Here's how the part is built. I have some questions about the finished solid (model axes, mm). Face numbers are marked on the shaded views. A direction names the side the tool comes from. Round coordinates to 2 decimals unless told otherwise and drop trailing zeros. Write each loop counter-clockwise with the first axis right and the second up, starting at its lowest first coordinate (ties: lowest second). Pieces come first, ordered by that corner, then holes. Notation, with made-up numbers: (7, 81) - (45, 81) arc R24 cw to (45, 119) - close; hole circle Ø6 at (-8.75, 80.25). An arc over 180 degrees is marked (long way). One line per item, written item: value. Start each with the question number.
Item 1: Thinking about a two-plate mould opening in X: for the marked faces 3, 4 and 5, which applies, released by +X, released by -X, zero draft, split by the parting line, or undercut?
Item 2: Imagine slicing it at C-C, the plane y = -70. Please give me the cut outline in (x, z), then the cut area to 3 significant figures.
Item 3: Imagine slicing it at B-B, the plane z = -74.5. Please give me the cut outline in (x, y).
Item 4: Imagine slicing it at D-D, the plane z = -63. Please give me the cut outline in (x, y), then the cut area to 3 significant figures.
Item 5: For P1, Ø3.5, axis at y = 11.5, z = -28.5, coming from the -X side; P2, Ø3, axis at x = 11.5, y = -166.5, coming from the +Z side; P3, Ø3.5, axis at y = 15.27, z = -50, coming from the +X side; P4, Ø8, axis at x = 19.5, z = -19.5, coming from the +Y side, each with a flat end and sliding along its axis, tell me the tip position at first contact or that it passes through.
Item 6: For the marked faces 1 and 2, which set-ups out of +Z, -Z, +X, -X, +Y, -Y let a thin tool reach every point of the face, with its end or its side?
Item 7: Imagine slicing it at A-A, the plane z = -39. Please give me the cut outline in (x, y).
Item 8: If I drill on line 1 (X direction, y = -7, z = -71); line 2 (X direction, y = -242.6, z = -4.5); line 3 (X direction, y = -131.5, z = -14), over which ranges is the centre line in solid material (lowest first)?
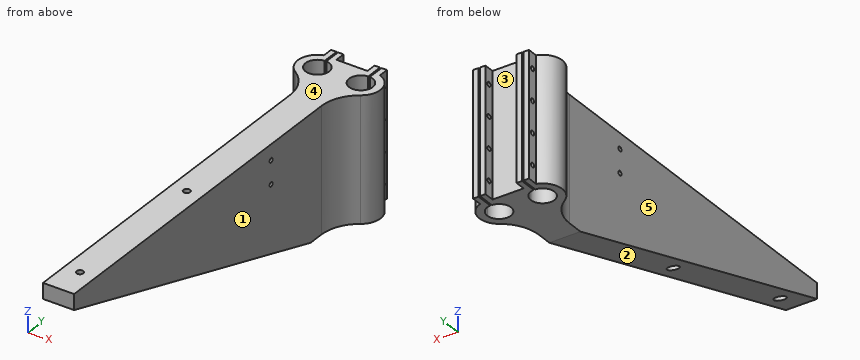
```python
from build123d import *

# Parameters (mm, degrees)
F0_R      = 7.6
F1_DEPTH  = 80
F2_DEPTH  = 80
F3_R      = 2.15
F4_DEPTH  = 80.001
F5_R      = 3.65
F6_DEPTH  = 70
F8_DEPTH  = 36.601
F9_W      = 0.5
F9_H      = 18.6
F10_DEPTH = 80.001
F11_R     = 1.45
F12_DEPTH = 44.601
F13_R     = 1.45
F14_DEPTH = 36.601


with BuildPart() as f1:
    # F0 (on Top) → F1 (new body)
    with BuildSketch(Plane.XY):
        with BuildLine():
            Line((-4, 18.6), (-4, 11.948222))
            ThreePointArc((-4, 11.948222), (-12.485747, 1.692961), (-7.037234, -10.451667))
            ThreePointArc((-7.037234, -10.451667), (1.06886, -19.443232), (4, -31.189101))
            Line((4, -31.189101), (4, -262.6))
            Line((4, -262.6), (24, -262.6))
            Line((24, -262.6), (24, -31.189101))
            ThreePointArc((24, -31.189101), (26.93114, -19.443232), (35.037234, -10.451667))
            ThreePointArc((35.037234, -10.451667), (40.485747, 1.692961), (32, 11.948222))
            Line((32, 11.948222), (32, 18.6))
            Line((32, 18.6), (24, 18.6))
            Line((24, 18.6), (24, 11.948222))
            Line((24, 11.948222), (4, 11.948222))
            Line((4, 11.948222), (4, 18.6))
            Line((4, 18.6), (-4, 18.6))
        make_face()
        Circle(F0_R, mode=Mode.SUBTRACT)
        with Locations((28, 0)):
            Circle(F0_R, mode=Mode.SUBTRACT)
    extrude(amount=-F1_DEPTH)

    # F0 (on Top) → F2 (join)
    with BuildSketch(Plane.XY):
        with BuildLine():
            Line((-4, 18.6), (-4, 11.948222))
            ThreePointArc((-4, 11.948222), (-12.485747, 1.692961), (-7.037234, -10.451667))
            ThreePointArc((-7.037234, -10.451667), (1.06886, -19.443232), (4, -31.189101))
            Line((4, -31.189101), (4, -262.6))
            Line((4, -262.6), (24, -262.6))
            Line((24, -262.6), (24, -31.189101))
            ThreePointArc((24, -31.189101), (26.93114, -19.443232), (35.037234, -10.451667))
            ThreePointArc((35.037234, -10.451667), (40.485747, 1.692961), (32, 11.948222))
            Line((32, 11.948222), (32, 18.6))
            Line((32, 18.6), (24, 18.6))
            Line((24, 18.6), (24, 11.948222))
            Line((24, 11.948222), (4, 11.948222))
            Line((4, 11.948222), (4, 18.6))
            Line((4, 18.6), (-4, 18.6))
        make_face()
        Circle(F0_R, mode=Mode.SUBTRACT)
        with Locations((28, 0)):
            Circle(F0_R, mode=Mode.SUBTRACT)
    extrude(amount=-F2_DEPTH)

    # F3 (on face) → F4 (cut, through all)
    with BuildSketch(Plane.XY):
        with Locations((14, -142.6)):
            Circle(F3_R)
        with Locations((14, -242.6)):
            Circle(F3_R)
    extrude(amount=-F4_DEPTH, mode=Mode.SUBTRACT)

    # F5 (on face) → F6 (cut)
    with BuildSketch(Plane(origin=(0, 0, -80), x_dir=(1, 0, 0), z_dir=(0, 0, -1))):
        with Locations((14, 242.6)):
            Circle(F5_R)
        with Locations((14, 142.6)):
            Circle(F5_R)
    extrude(amount=-F6_DEPTH, mode=Mode.SUBTRACT)

    # F7 (on face) → F8 (cut, through all)
    with BuildSketch(Plane(origin=(4, 0, 0), x_dir=(0, -1, 0), z_dir=(-1, 0, 0))):
        Polygon((262.6, -80), (262.6, -10), (41.189101, -80), align=None)
    extrude(amount=-F8_DEPTH, mode=Mode.SUBTRACT)

    # F9 (on face) → F10 (cut, through all)
    with BuildSketch(Plane.XY):
        with Locations((-0.25, 9.3)):
            Rectangle(F9_W, F9_H)
        with Locations((0.25, 9.3)):
            Rectangle(F9_W, F9_H)
        with Locations((27.75, 9.3)):
            Rectangle(F9_W, F9_H)
        with Locations((28.25, 9.3)):
            Rectangle(F9_W, F9_H)
    extrude(amount=-F10_DEPTH, mode=Mode.SUBTRACT)

    # F11 (on face) → F12 (cut, through all)
    with BuildSketch(Plane(origin=(-4, 0, 0), x_dir=(0, -1, 0), z_dir=(-1, 0, 0))):
        with Locations((-15.274111, -30)):
            Circle(F11_R)
        with Locations((-15.274111, -70)):
            Circle(F11_R)
        with Locations((-15.274111, -50)):
            Circle(F11_R)
        with Locations((-15.274111, -10)):
            Circle(F11_R)
    extrude(amount=-F12_DEPTH, mode=Mode.SUBTRACT)

    # F13 (on face) → F14 (cut, through all)
    with BuildSketch(Plane(origin=(4, 0, 0), x_dir=(0, -1, 0), z_dir=(-1, 0, 0))):
        with Locations((78.189101, -10)):
            Circle(F13_R)
        with Locations((78.189101, -25)):
            Circle(F13_R)
    extrude(amount=-F14_DEPTH, mode=Mode.SUBTRACT)


solid = f1.part
```
Values follow:
1. face 3: undercut
1. face 4: zero draft
1. face 5: released by -X
2. outline: (4, -70.89) - (24, -70.89) - (24, 0) - (4, 0) - close
2. area: 1,420 mm^2
3. outline: (-7.04, -10.45) arc R25 cw to (4, -31.19) - (4, -58.59) - (24, -58.59) - (24, -31.19) arc R25 cw to (35.04, -10.45) arc R12.6 ccw to (32, 11.95) - (32, 18.6) - (28.5, 18.6) - (28.5, 7.58) arc R7.6 cw (long way) to (27.5, 7.58) - (27.5, 18.6) - (24, 18.6) - (24, 11.95) - (4, 11.95) - (4, 18.6) - (0.5, 18.6) - (0.5, 7.58) arc R7.6 cw (long way) to (-0.5, 7.58) - (-0.5, 18.6) - (-4, 18.6) - (-4, 11.95) arc R12.6 ccw to start
4. outline: (-7.04, -10.45) arc R25 cw to (4, -31.19) - (4, -94.96) - (24, -94.96) - (24, -31.19) arc R25 cw to (35.04, -10.45) arc R12.6 ccw to (32, 11.95) - (32, 18.6) - (28.5, 18.6) - (28.5, 7.58) arc R7.6 cw (long way) to (27.5, 7.58) - (27.5, 18.6) - (24, 18.6) - (24, 11.95) - (4, 11.95) - (4, 18.6) - (0.5, 18.6) - (0.5, 7.58) arc R7.6 cw (long way) to (-0.5, 7.58) - (-0.5, 18.6) - (-4, 18.6) - (-4, 11.95) arc R12.6 ccw to start
4. area: 2,650 mm^2
5. P1: stops at x = -7.98
5. P2: stops at z = 0
5. P3: stops at x = 32
5. P4: stops at y = 11.95
6. face 1: +Z, -Z, +X, -Y
6. face 2: -Z, +X, -X, -Y
7. outline: (-7.04, -10.45) arc R25 cw to (4, -31.19) - (4, -170.87) - (24, -170.87) - (24, -31.19) arc R25 cw to (35.04, -10.45) arc R12.6 ccw to (32, 11.95) - (32, 18.6) - (28.5, 18.6) - (28.5, 7.58) arc R7.6 cw (long way) to (27.5, 7.58) - (27.5, 18.6) - (24, 18.6) - (24, 11.95) - (4, 11.95) - (4, 18.6) - (0.5, 18.6) - (0.5, 7.58) arc R7.6 cw (long way) to (-0.5, 7.58) - (-0.5, 18.6) - (-4, 18.6) - (-4, 11.95) arc R12.6 ccw to start; hole circle Ø7.3 at (14, -142.6)
8. line 1: x = -10.48 to -2.96, 2.96 to 25.04, 30.96 to 38.48
8. line 2: x = 4 to 11.85, 16.15 to 24
8. line 3: x = 4 to 24
